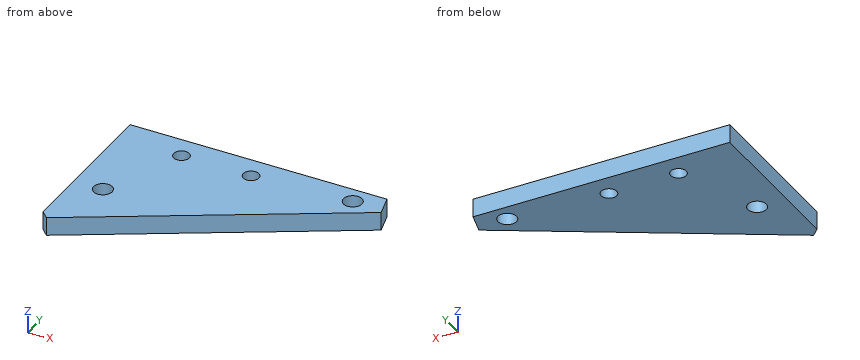
from build123d import *

# Parameters (mm, degrees)
BOSS_EXTRUDE1_DEPTH    = 3.175
M2_5_CLEARANCE_HOLE1_D = 2.7
CHAMFER1_SIZE          = 2
CHAMFER1_SIZE2         = 1.464101615
M3_CLEARANCE_HOLE1_D   = 3.2


with BuildPart() as part:
    # Sketch2 → Boss-Extrude1 (new body)
    with BuildSketch(Plane.XY):
        Polygon((17, 4), (-17, 4), (-17, -25.879909152), (34.753520778, 4), align=None)
    extrude(amount=BOSS_EXTRUDE1_DEPTH)

    # M2.5 Clearance Hole1 (through all)
    with Locations(Plane.XY.offset(3.175)):
        with Locations((-6, 0), (6, 0)):
            Hole(M2_5_CLEARANCE_HOLE1_D / 2)

    # Fillet1
    # the kernel refuses this chamfer: 2 mm, written as the material it takes off along each edge
    with BuildSketch(Plane(origin=(34.753520778, 4, -18.713015054), x_dir=(-0.9999467105068274, 0.01032357237467217, 0), z_dir=(0, 0, 1))) as fillet1_piece_1:
        with BuildLine():
            Line((7.485206022, 0), (6.403726885, 3.875640743))
            Line((6.403726885, 3.875640743), (6.383370332, 3.910073441))
            ThreePointArc((6.383370332, 3.910073441), (3.20116981, 1.938993637), (-0.020356553, 0.034432699))
            Line((-0.020356553, 0.034432699), (0.000412943, -0.039997868))
            ThreePointArc((0.000412943, -0.039997868), (3.742617081, -0.001362894), (7.485618964, -0.039997868))
            Line((7.485618964, -0.039997868), (7.485206022, 0))
        make_face()
    extrude(amount=40.601030108, mode=Mode.SUBTRACT)

    # Chamfer1
    chamfer1_edges = [part.edges().sort_by_distance(p)[0] for p in [
        (-17, -25.879909152, 1.5875),
    ]]
    chamfer1_side = [part.faces().sort_by_distance(p)[0] for p in [
        (-17, -10.939954576, 1.5875),
    ]]
    chamfer(chamfer1_edges, length=CHAMFER1_SIZE, length2=CHAMFER1_SIZE2, reference=chamfer1_side[0])

    # M3 Clearance Hole1 (through all)
    with Locations(Plane(origin=(0, 0, 0), x_dir=(-1, 0, 0), z_dir=(0, 0, -1))):
        with Locations((-23, 1), (12, -14)):
            Hole(M3_CLEARANCE_HOLE1_D / 2)


solid = part.part
Design review of the part built by this model. Coordinates are the model's own, in mm. Round coordinates to 2 decimals unless told otherwise and drop trailing zeros. Write each loop counter-clockwise with the first axis right and the second up, starting at its lowest first coordinate (ties: lowest second). Pieces come first, ordered by that corner, then holes.
Item 1: Consider section A-A on z = 1.5. Give the boundary of the cut face in (x, y).
Item 2: Wall thickness on L1, parallel to X at y = 0.5, z = 1; L2, parallel to X at y = 2.25, z = 1.95; L3, parallel to Y at x = 6, z = 1.8: over which ranges is each line inside the solid? List them lowest first.
Item 3: Consider section D-D on x = 0. Give the boundary of the cut face in (y, z) (3 decimals), and give its area (3 significant figures).
Item 4: Consider section C-C on y = -14. Give the boundary of the cut face in (x, z) (3 decimals).
Item 5: For pin 1 Ø1 at (x, z) = (-12, 2.5) entering from -Y, flat-tipped, find the tip position at first contact; note if it passes through.
Item 6: Consider section B-B on x = 23. Give the boundary of the cut face in (y, z) (3 decimals).
Check values:
1. outline: (-17, -23.88) - (-15.73, -25.15) - (28.29, 0.27) - (27.29, 4) - (-17, 4) - close; hole circle Ø3.2 at (-12, -14); hole circle Ø2.7 at (-6, 0); hole circle Ø2.7 at (6, 0); hole circle Ø3.2 at (23, 1)
2. L1: x = -17 to -7.25, -4.75 to 4.75, 7.25 to 21.48, 24.52 to 28.23
2. L2: x = -17 to 22, 24 to 27.76
2. L3: y = -12.6 to -1.35, 1.35 to 4
3. outline: (-16.065, 0) - (4, 0) - (4, 3.175) - (-16.065, 3.175) - close
3. area: 63.7 mm2
4. outline: (-17, 0) - (-13.6, 0) - (-13.6, 3.175) - (-17, 3.175) - close; (-10.4, 0) - (3.577, 0) - (3.577, 3.175) - (-10.4, 3.175) - close
5. pin 1: stops at y = -23.28
6. outline: (-2.786, 0) - (-0.6, 0) - (-0.6, 3.175) - (-2.786, 3.175) - close; (2.6, 0) - (4, 0) - (4, 3.175) - (2.6, 3.175) - close
